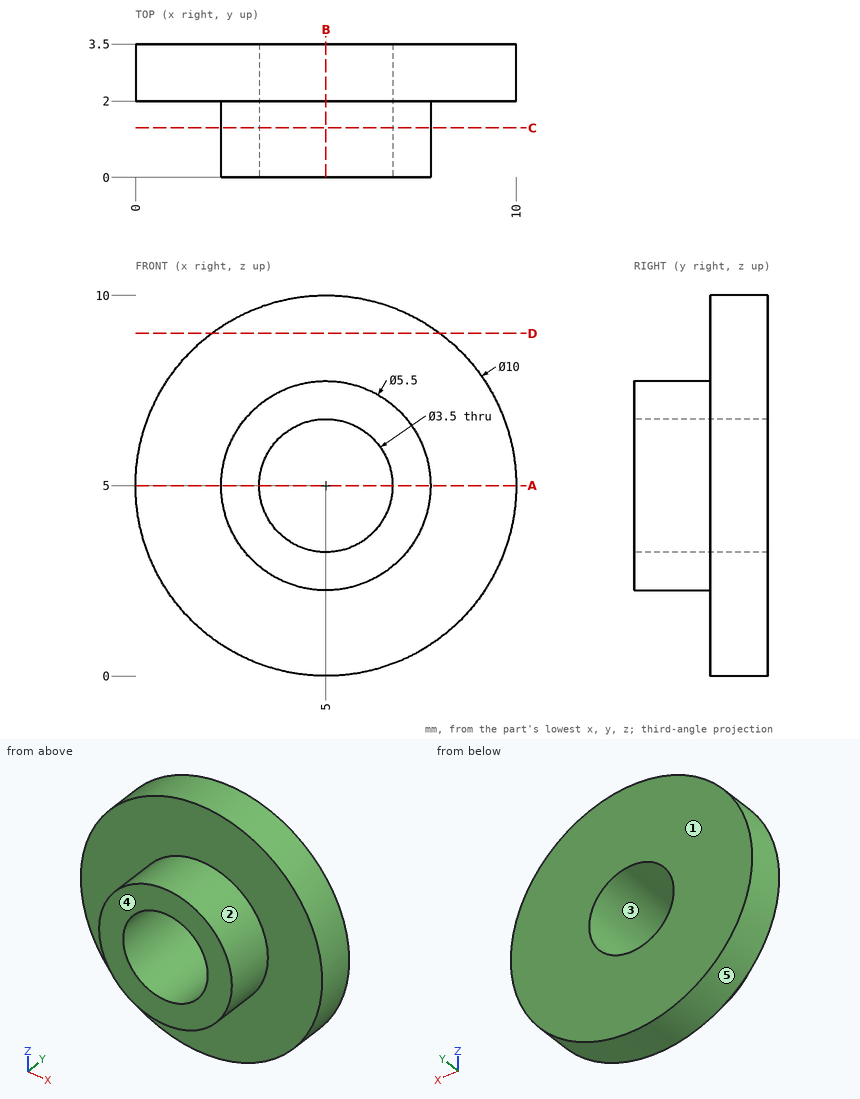
Verification items for this drawing (mm, ordinates from the low corner). A direction names the side the tool comes from. Coordinates: 2 decimals unless noted, no trailing zeros. Loops run counter-clockwise (first coordinate to the right, second up) from the corner with the lowest first, then second, coordinate; pieces in that order, holes last. Notation, with made-up numbers: (-1, 37) -> (52, 37) arc R22 ccw to (52, 56) -> close; hole circle Ø4 at (88, 72). An arc over 180 degrees is marked (long way). Put each result on its own line as item: value.
1. Gauge pin test, flat ends, axial feed: P1, Ø3, axis at x = 5, z = 5, coming from the -Y side; P2, Ø1, axis at y = 2, z = 6.5, coming from the -X side; P3, Ø1, axis at y = 0.5, z = 2, coming from the +X side. Record the tip position at first contact, or that the pin passes through.
Result set:
P1: passes through
P2: stops at x = 0.1
P3: stops at x = 6.15
2. Tool access check on the marked faces 1 and 2. Record the directions out of +Z, -Z, +X, -X, +Y, -Y that give a thin tool (end or side, any length) a straight path to the whole face; none if there is none.
Result set:
face 1: +Z, -Z, +X, -X, +Y
face 2: -Y
3. Thickness scan on line 1 (Z direction, x = 5, y = 1.2); line 2 (Z direction, x = 5, y = 2.1). Record the ranges inside material, lowest first.
Result set:
line 1: z = 2.25 to 3.25, 6.75 to 7.75
line 2: z = 0 to 3.25, 6.75 to 10
4. Section check A-A, the plane z = 5. Record the boundary of the cut face in (x, y).
Result set:
outline: (0, 2) -> (2.25, 2) -> (2.25, 0) -> (3.25, 0) -> (3.25, 3.5) -> (0, 3.5) -> close; (6.75, 0) -> (7.75, 0) -> (7.75, 2) -> (10, 2) -> (10, 3.5) -> (6.75, 3.5) -> close
5. Section check C-C, the plane y = 1.3. Record the boundary of the cut face in (x, z), then the cut area to 3 significant figures.
Result set:
outline: circle Ø5.5 at (5, 5); hole circle Ø3.5 at (5, 5)
area: 14.1 mm^2
6. Section check D-D, the plane z = 9. Record the boundary of the cut face in (x, y), then the cut area to 3 significant figures.
Result set:
outline: (2, 2) -> (8, 2) -> (8, 3.5) -> (2, 3.5) -> close
area: 9.00 mm^2
7. Mould release check, pull along X, two halves, no side actions. Record for the marked faces 3, 4 and 5: pulls with the +X half, pulls with the -X half, needs draft (parallel to the pull), parting line crosses it, or undercut.
Result set:
face 3: undercut
face 4: needs draft
face 5: parting line crosses it
8. Section check B-B, the plane x = 5. Record the boundary of the cut face in (y, z).
Result set:
outline: (0, 2.25) -> (2, 2.25) -> (2, 0) -> (3.5, 0) -> (3.5, 3.25) -> (0, 3.25) -> close; (0, 6.75) -> (3.5, 6.75) -> (3.5, 10) -> (2, 10) -> (2, 7.75) -> (0, 7.75) -> close
